from build123d import *

# Parameters (mm, degrees)
PAD002_DEPTH   = 16
SKETCH005_R    = 3.3
HOLE002_DEPTH  = 6
HOLE002_TIPS_R = 3.3


with BuildPart() as part:
    # Sketch004 → Pad002 (new body)
    with BuildSketch(Plane.XY):
        Polygon((-5, 3), (5, 3), (8, 0), (8, -1.2), (3.9, -1.2), (3.9, -3), (-3.9, -3), (-3.9, -1.2), (-8, -1.2), (-8, 0), align=None)
    extrude(amount=PAD002_DEPTH)

    # Sketch005 (on Face6 of Pad002) → Hole002 (cut)
    with BuildSketch(Plane.XZ.offset(3)):
        with Locations((0, 8)):
            Circle(SKETCH005_R)
    extrude(amount=-HOLE002_DEPTH, mode=Mode.SUBTRACT)

    # Hole002 tips → Hole002 tip 1 section 0
    with BuildSketch(Plane.XZ.offset(-3), mode=Mode.PRIVATE) as hole002_tip_1_s0:
        with Locations((0, 8)):
            Circle(HOLE002_TIPS_R)
    loft([hole002_tip_1_s0.sketch, Vertex(0, 4.98284, 8)], mode=Mode.SUBTRACT)


solid = part.part
Can you work these out from the model? Positions are in its coordinate system, mm. A direction names the side the tool comes from. Give positions to 0.01 mm unless a question says otherwise; leave off trailing zeros. Loops run counter-clockwise (first coordinate to the right, second up) from the corner with the lowest first, then second, coordinate; pieces in that order, holes last. Notation, with made-up numbers: (89, -34) -> (125, -34) arc R17 ccw to (125, -25) -> close; hole circle Ø2 at (18, -21.5). An arc over 180 degrees is marked (long way). Return JSON: item names as keys, results as strings.
Q1. For pin 1 Ø4.5 at (x, z) = (-6.5, 12) entering from -Y; pin 2 Ø0.9 at (y, z) = (-2, 8) entering from +X; pin 3 Ø0.9 at (y, z) = (-2, 6.5) entering from -X, each with a flat end and sliding along its axis, tell me the tip position at first contact or that it passes through.
Checks:
{"pin 1": "stops at y = -1.2", "pin 2": "stops at x = 3.9", "pin 3": "stops at x = -3.9"}
Q2. I want a section at B-B, the plane y = -1.85. List the corners of the cut face in (x, z) for me.
Checks:
{"outline": "(-3.9, 0) -> (3.9, 0) -> (3.9, 16) -> (-3.9, 16) -> close; hole circle Ø6.6 at (0, 8)"}
Q3. I want a section at A-A, the plane x = 0. List the corners of the cut face in (y, z) for me.
Checks:
{"outline": "(-3, 0) -> (3, 0) -> (3, 4.7) -> (-3, 4.7) -> close; (-3, 11.3) -> (3, 11.3) -> (3, 16) -> (-3, 16) -> close"}
Q4. I want a section at C-C, the plane z = 8. List the corners of the cut face in (x, y) for me, then the cut area to 3 significant figures.
Checks:
{"outline": "(-8, -1.2) -> (-3.9, -1.2) -> (-3.9, -3) -> (-3.3, -3) -> (-3.3, 3) -> (-5, 3) -> (-8, 0) -> close; (3.3, -3) -> (3.9, -3) -> (3.9, -1.2) -> (8, -1.2) -> (8, 0) -> (5, 3) -> (3.3, 3) -> close", "area": "32.6 mm2"}
Q5. We'd pull the mould along X, two halves only. Please class faces 1 (the face through (0, 0, 0)), 2 (the face through (-0.72, -0.04, 4.78)), 3 (the face through (-8, -1, 8)): released by +X, released by -X, zero draft, split by the parting line, or undercut.
Checks:
{"face 1": "zero draft", "face 2": "undercut", "face 3": "released by -X"}
Q6. On a 3-axis mill with a long thin cutter (end or side, diameter ignored), from which of +Z, -Z, +X, -X, +Y, -Y can I reach the whole of each face in a straight line? I mean faces 4 (the face through (0, 0, 16)), 5 (the face through (-3.9, -2, 8)), 6 (the face through (6, -1.2, 8)). Say none if no direction works.
Checks:
{"face 4": "+Z, +X, -X, +Y, -Y", "face 5": "+Z, -Z, -X, -Y", "face 6": "+Z, -Z, +X, -Y"}
Q7. I want a section at D-D, the plane z = 2.5. List the corners of the cut face in (x, y) for me.
Checks:
{"outline": "(-8, -1.2) -> (-3.9, -1.2) -> (-3.9, -3) -> (3.9, -3) -> (3.9, -1.2) -> (8, -1.2) -> (8, 0) -> (5, 3) -> (-5, 3) -> (-8, 0) -> close"}
Q8. I need wall thicknesses on probe 1 along Z at (x, y) = (0, 0.6); probe 2 along X at (y, z) = (0.1, 8.5); probe 3 along X at (y, z) = (-2.6, 15.5). Which ranges of each line are inside material? Lowest first, please.
Checks:
{"probe 1": "z = 0 to 4.7, 11.3 to 16", "probe 2": "x = -7.9 to -3.26, 3.26 to 7.9", "probe 3": "x = -3.9 to 3.9"}
